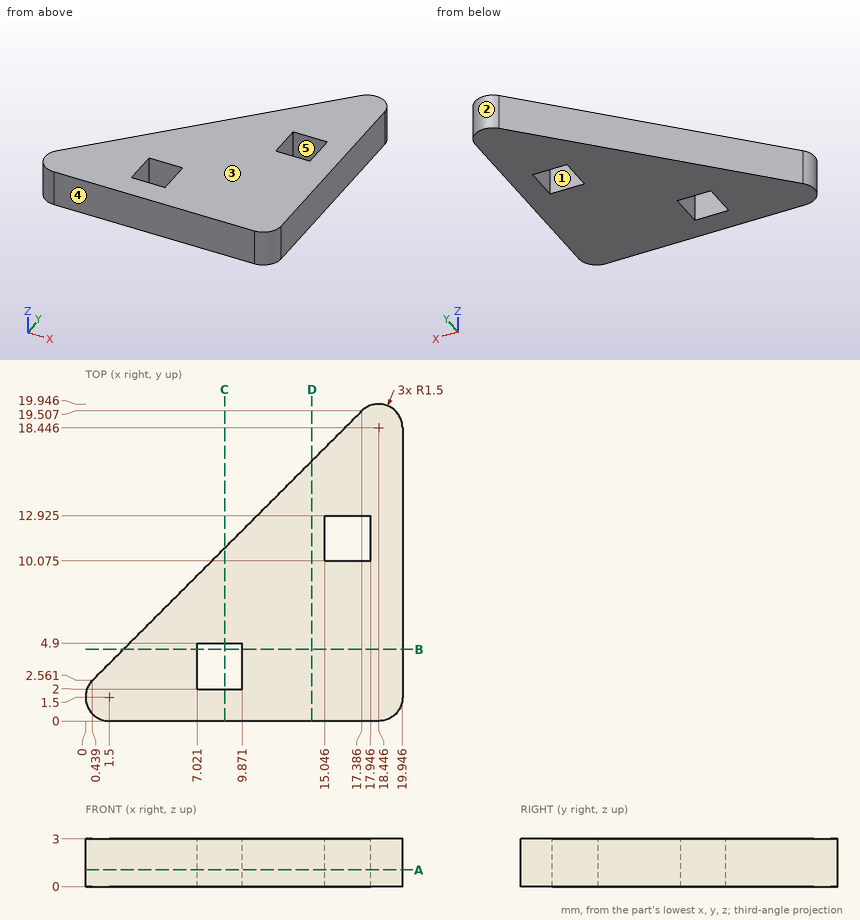
Study the drawing (mm; zero at the part's minimum x, y, z) and answer. A direction names the side the tool comes from. Coordinates: 2 decimals unless noted, no trailing zeros. Write each loop counter-clockwise with the first axis right and the second up, starting at its lowest first coordinate (ties: lowest second). Pieces come first, ordered by that corner, then holes. Notation, with made-up numbers: (-38.5, 26) - (-14.5, 26) arc R30 ccw to (-14.5, 62) - close; hole circle Ø2 at (23.25, -12.5). An arc over 180 degrees is marked (long way). Return JSON: item names as keys, results as strings. Group by question number.
1. A cutting plane is placed at D-D, the plane x = 14.25. Determine the outline of the cut face in (y, z), plus the area to 3 significant figures.
2. Given pin 1 (1 mm diameter, centred on x = 4, z = 2.5, fed in from +Y); pin 2 (0.9 mm diameter, centred on y = 11.5, z = 1.5, fed in from -X); pin 3 (1.5 mm diameter, centred on x = 11.5, z = 1, fed in from +Y), each flat-ended and moving along its own axis, determine where each tip first touches the part or whether it passes through.
3. Determine the mould class of the marked faces 3, 4 and 5 for opening direction Y: released by +Y, released by -Y, zero draft, split by the parting line, or undercut.
4. A cutting plane is placed at C-C, the plane x = 8.75. Determine the outline of the cut face in (y, z).
5. A cutting plane is placed at A-A, the plane z = 1.05. Determine the outline of the cut face in (x, y) (1 decimal), plus the area to 3 significant figures.
6. Straight lines are drawn through the part: L1, parallel to X at y = 4.5, z = 0.8 (1 decimal); L2, parallel to Y at x = 16.25, z = 0.45 (1 decimal); L3, parallel to X at y = 4, z = 2.7 (1 decimal). For each, find the intervals that lie inside material, in ascending order.
7. A cutting plane is placed at B-B, the plane y = 4.5. Determine the outline of the cut face in (x, z).
8. Which of the six approach directions +Z, -Z, +X, -X, +Y, -Y give full straight-line access (tool end or side, diameter ignored) to the marked faces 1 and 2?
Ans:
{
 "1": {"outline": "(0, 0) - (16.37, 0) - (16.37, 3) - (0, 3) - close", "area": "49.1 mm²"},
 "2": {"pin 1": "y = 6.62", "pin 2": "x = 8.93", "pin 3": "y = 14.37"},
 "3": {"face 3": "zero draft", "face 4": "released by -Y", "face 5": "undercut"},
 "4": {"outline": "(0, 0) - (2, 0) - (2, 3) - (0, 3) - close; (4.9, 0) - (10.87, 0) - (10.87, 3) - (4.9, 3) - close"},
 "5": {"outline": "(0.4, 2.6) arc R1.5 ccw to (1.5, 0) - (18.4, 0) arc R1.5 ccw to (19.9, 1.5) - (19.9, 18.4) arc R1.5 ccw to (17.4, 19.5) - close; hole (7, 2) - (9.9, 2) - (9.9, 4.9) - (7, 4.9) - close; hole (15, 10.1) - (17.9, 10.1) - (17.9, 12.9) - (15, 12.9) - close", "area": "221 mm²"},
 "6": {"L1": "2.4 to 7, 9.9 to 19.9", "L2": "0 to 10.1, 12.9 to 18.4", "L3": "1.9 to 7, 9.9 to 19.9"},
 "7": {"outline": "(2.38, 0) - (7.02, 0) - (7.02, 3) - (2.38, 3) - close; (9.87, 0) - (19.95, 0) - (19.95, 3) - (9.87, 3) - close"},
 "8": {"face 1": "+Z, -Z", "face 2": "+Z, -Z, +Y"}
}
